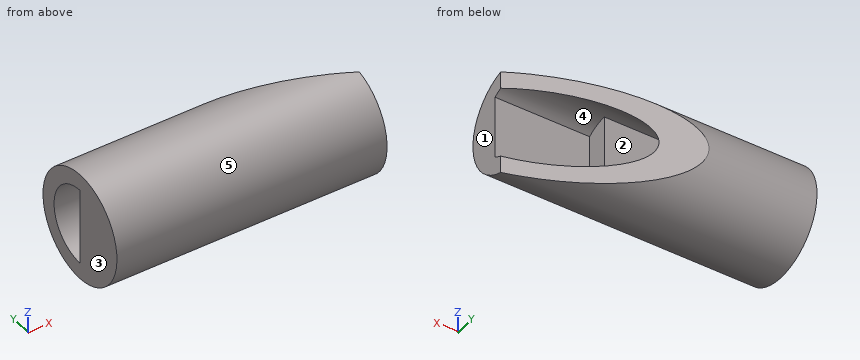
from build123d import *

# Parameters (mm, degrees)
BOSS_EXTRUDE1_DEPTH            = 65
SKETCH1_4_R                    = 20
SKETCH1_4_R_2                  = 14
BOSS_EXTRUDE2_DEPTH            = 100
CUT_EXTRUDE1_REACH             = 105.923
CUT_EXTRUDE1_DIRECTION_2_REACH = 105.923


with BuildPart() as part:
    # Sketch1 → Boss-Extrude1 (new body)
    with BuildSketch(Plane(origin=(0, 0, 0), x_dir=(0, 0, -1), z_dir=(1, 0, 0))):
        with BuildLine():
            Line((14, 0), (-14, 0))
            ThreePointArc((-14, 0), (-13.357540082, -4.192388692), (-11.489125293, -8))
            Line((-11.489125293, -8), (11.489125293, -8))
            ThreePointArc((11.489125293, -8), (13.357540082, -4.192388692), (14, 0))
        make_face()
    extrude(amount=BOSS_EXTRUDE1_DEPTH)

    # Sketch1_4 → Boss-Extrude2 (add)
    # profile 1 of 2: a face of its own
    with BuildSketch(Plane(origin=(0, 0, 0), x_dir=(0, 0, -1), z_dir=(1, 0, 0))):
        Circle(SKETCH1_4_R)
        Circle(SKETCH1_4_R_2, mode=Mode.SUBTRACT)
    # profile 2 of 2: a face of its own
    with BuildSketch(Plane(origin=(0, 0, 0), x_dir=(0, 0, -1), z_dir=(1, 0, 0))):
        with BuildLine():
            Line((11.489125293, -8), (-11.489125293, -8))
            ThreePointArc((-11.489125293, -8), (0, -14), (11.489125293, -8))
        make_face()
    extrude(amount=BOSS_EXTRUDE2_DEPTH)

    # Sketch2 → Cut-Extrude1 (cut, up to next)
    with BuildSketch(Plane.XY, mode=Mode.PRIVATE) as cut_extrude1_sk1:
        Polygon((40, 20), (100, -5), (100, 20), align=None)
    cut_extrude1_tool1 = extrude(cut_extrude1_sk1.sketch, amount=-CUT_EXTRUDE1_REACH, mode=Mode.PRIVATE) & part.part
    add(cut_extrude1_tool1.solids().sort_by_distance((80, 11.666667, 0))[0], mode=Mode.SUBTRACT)

    # Sketch2 → Cut-Extrude1 direction 2 (cut, up to next)
    with BuildSketch(Plane.XY, mode=Mode.PRIVATE) as cut_extrude1_direction_2_sk1:
        Polygon((40, 20), (100, -5), (100, 20), align=None)
    cut_extrude1_direction_2_tool1 = extrude(cut_extrude1_direction_2_sk1.sketch, amount=CUT_EXTRUDE1_DIRECTION_2_REACH, mode=Mode.PRIVATE) & part.part
    add(cut_extrude1_direction_2_tool1.solids().sort_by_distance((80, 11.666667, 0))[0], mode=Mode.SUBTRACT)


solid = part.part
Can you work these out from the model? Positions are in its coordinate system, mm. Face numbers are marked on the shaded views. A direction names the side the tool comes from. Coordinates: 2 decimals unless noted, no trailing zeros. Write each loop counter-clockwise with the first axis right and the second up, starting at its lowest first coordinate (ties: lowest second). Pieces come first, ordered by that corner, then holes. Notation, with made-up numbers: (41, 55.25) -> (79, 55.25) arc R15 ccw to (79, 74.25) -> close; hole circle Ø1 at (87.5, -26). An arc over 180 degrees is marked (long way). Write item = value, one per line.
(1) Imagine slicing it at C-C (x = 27.5). Please give me the cut outline in (y, z).
Verdict:
outline = circle Ø40 at (0, 0); hole (0, -14) arc R14 ccw to (0, 14) -> close
(2) If I drill on probe 1 along Y at (x, z) = (37.5, 0); probe 2 along X at (y, z) = (-1, -8.5); probe 3 along Z at (x, y) = (74, 2), over which ranges is the centre line in solid material (lowest first)?
Verdict:
probe_1 = -20 to 0, 14 to 20
probe_2 = 0 to 65
probe_3 = -19.9 to -13.86, 13.86 to 19.9
(3) Thinking about a two-plate mould opening in Z: for the marked faces 3, 4 and 5, which applies, +Z half, -Z half, draft (parallel to the pull), parting line (faces both ways), or undercut?
Verdict:
face_3 = draft
face_4 = undercut
face_5 = parting line
(4) Imagine slicing it at B-B (y = 9.5). Please give me the cut outline in (x, z).
Verdict:
outline = (0, -17.6) -> (65.2, -17.6) -> (65.2, -10.28) -> (0, -10.28) -> close; (0, 10.28) -> (65.2, 10.28) -> (65.2, 17.6) -> (0, 17.6) -> close
(5) Imagine slicing it at D-D (y = -1). Please give me the cut outline in (x, z), and give its area (3 significant figures).
Verdict:
outline = (0, -19.97) -> (90.4, -19.97) -> (90.4, -13.96) -> (65, -13.96) -> (65, 13.96) -> (90.4, 13.96) -> (90.4, 19.97) -> (0, 19.97) -> close
area = 2,900 mm^2
(6) For pin 1 (5 mm diameter, centred on x = 87.5, z = -3.5, fed in from -Y) (3 decimals); pin 2 (12 mm diameter, centred on x = 40, z = -10, fed in from +Y); pin 3 (3 mm diameter, centred on x = 75, z = 12.5, fed in from -Y), each with a flat end and sliding along its axis, tell me the tip position at first contact or that it passes through.
Verdict:
pin_1 = -19.975
pin_2 = 19.6
pin_3 = -16.7
(7) Imagine slicing it at A-A (z = 0). Please give me the cut outline in (x, y), and give its area (3 significant figures).
Verdict:
outline = (0, -20) -> (100, -20) -> (100, -8) -> (65, -8) -> (65, 0) -> (0, 0) -> close; (0, 14) -> (54.4, 14) -> (40, 20) -> (0, 20) -> close
area = 2,000 mm^2
(8) On a 3-axis mill with a long thin cutter (end or side, diameter ignored), from which of +Z, -Z, +X, -X, +Y, -Y can I reach the whole of each face in a straight line? I mean the marked faces 1 and 2. Say none if no direction works.
Verdict:
face_1 = +Z, -Z, +X, +Y, -Y
face_2 = +X, -X
